Design review of the part built by this model. Coordinates are the model's own, in mm. A direction names the side the tool comes from. Round coordinates to 2 decimals unless told otherwise and drop trailing zeros. Loops run counter-clockwise (first coordinate to the right, second up) from the corner with the lowest first, then second, coordinate; pieces in that order, holes last. Notation, with made-up numbers: (51.25, 21) -> (103.25, 21) arc R21 ccw to (103.25, 39) -> close; hole circle Ø8 at (86.5, 81.5). An arc over 180 degrees is marked (long way). Write each question's results on one line, items separated by ' | '. Start each with the question number.
from build123d import *

# Parameters (mm, degrees)
ESQUISSE1_R                                = 1.4
BOSS_EXTRU_1_DEPTH                         = 6
ESQUISSE2_R                                = 3.25
ENL_V_MAT_EXTRU_1_DEPTH                    = 3
SYM_TRIE3_AT_THE_SECOND_PLANE_COPY_1_SKE_R = 3.25
SYM_TRIE3_AT_THE_SECOND_PLANE_COPY_1_DEPTH = 3
ESQUISSE4_W                                = 25
ESQUISSE4_H                                = 5
ESQUISSE4_W_2                              = 7.5
ESQUISSE4_H_2                              = 50
ENL_V_MAT_EXTRU_2_DEPTH                    = 102.655363655


with BuildPart() as part:
    # Esquisse1 → Boss.-Extru.1 (new body)
    with BuildSketch(Plane(origin=(0, 0, -27.5), x_dir=(-1, 0, 0), z_dir=(0, 0, -1))):
        Polygon((-2.565563678, -55.727752809), (62.179602326, -55.727752809), (84.807019324, -33.100335811), (84.807019324, 31.644830193), (62.179602326, 54.272247191), (-2.565563678, 54.272247191), (-25.192980676, 31.644830193), (-25.192980676, -33.100335811), align=None)
        with Locations((-9.63663149, 38.715898005)):
            Circle(ESQUISSE1_R, mode=Mode.SUBTRACT)
        with Locations((69.250670138, 38.715898005)):
            Circle(ESQUISSE1_R, mode=Mode.SUBTRACT)
        with Locations((69.250670138, -40.171403623)):
            Circle(ESQUISSE1_R, mode=Mode.SUBTRACT)
        with Locations((-9.63663149, -40.171403623)):
            Circle(ESQUISSE1_R, mode=Mode.SUBTRACT)
    extrude(amount=BOSS_EXTRU_1_DEPTH)

    # Esquisse2 → Enlèv. mat.-Extru.1 (cut)
    with BuildSketch(Plane(origin=(0, 0, -33.5), x_dir=(-1, 0, 0), z_dir=(0, 0, -1))):
        with Locations((69.250670138, 38.715898005)):
            Circle(ESQUISSE2_R)
    enl_v_mat_extru_1 = extrude(amount=-ENL_V_MAT_EXTRU_1_DEPTH, mode=Mode.SUBTRACT)

    # Symétrie3: Enlèv. mat.-Extru.1 across plane
    add(enl_v_mat_extru_1.mirror(Plane(origin=(-29.807019324, 0, 0), x_dir=(0, 0, 1), z_dir=(1, 0, 0))), mode=Mode.SUBTRACT)

    # Symétrie3 at the second plane: Enlèv. mat.-Extru.1 across plane
    add(enl_v_mat_extru_1.mirror(Plane(origin=(0, -0.727752809, 0), x_dir=(0, 0, 1), z_dir=(0, -1, 0))), mode=Mode.SUBTRACT)

    # Symétrie3 at the second plane copy 1 ske → Symétrie3 at the second plane copy 1 (cut)
    with BuildSketch(Plane(origin=(-59.614038648, -1.455505618, -33.5), x_dir=(1, 0, 0), z_dir=(0, 0, -1))):
        with Locations((69.250670138, 38.715898005)):
            Circle(SYM_TRIE3_AT_THE_SECOND_PLANE_COPY_1_SKE_R)
    extrude(amount=-SYM_TRIE3_AT_THE_SECOND_PLANE_COPY_1_DEPTH, mode=Mode.SUBTRACT)

    # Esquisse4 → Enlèv. mat.-Extru.2 (cut, through all)
    with BuildSketch(Plane(origin=(0, 0, -33.5), x_dir=(-1, 0, 0), z_dir=(0, 0, -1))):
        with Locations((39.250670138, -40.171403623)):
            Rectangle(ESQUISSE4_W, ESQUISSE4_H)
        with Locations((39.250670138, 38.715898005)):
            Rectangle(ESQUISSE4_W, ESQUISSE4_H)
        with Locations((-5.88663149, -0.727752809)):
            Rectangle(ESQUISSE4_W_2, ESQUISSE4_H_2)
    extrude(amount=-ENL_V_MAT_EXTRU_2_DEPTH, mode=Mode.SUBTRACT)


solid = part.part
1) Insertion check: pin 1 (7 mm diameter, centred on x = -70.5, y = -39.5, fed in from -Z); pin 2 (2.5 mm diameter, centred on x = -69.25, y = -40.17, fed in from +Z); pin 3 (2 mm diameter, centred on x = 9, y = -39, fed in from -Z); pin 4 (1.5 mm diameter, centred on y = 38, z = -30.5, fed in from -X). Each pin has a flat end and moves straight along its axis. Give the tip position at first contact, or say it passes through.
2) To check wall thickness, follow line 1 (Y direction, x = -32, z = -29.85); line 2 (X direction, y = 23, z = -31.6); line 3 (Y direction, x = -69, z = -31.1). State the ranges of each line that lie inside material, in increasing order. Write a range as from..to.
3) Take a section at A-A (y = 19). Write out the cut boundary in (x, z), plus the area to 3 significant figures.
4) For faces 4 (the face through (-39, -37.671, -31)), 5 (the face through (-72.35, -41.15, -32.02)), 6 (the face through (13.72, 43.12, -30.46)), list the 3-axis set-ups (+Z, -Z, +X, -X, +Y, -Y) from which the entire face can be reached by the end or side of a thin tool; tool diameter is ignored.
5) Take a section at C-C (z = -32.05). Write out the cut boundary in (x, y), plus the area to 3 significant figures.
6) The part is to be moulded in two halves that separate along X. For faces 1 (the face through (-51.751, -40, -31)), 2 (the face through (25.193, 0, -30)), 3 (the face through (-29, -55.728, -30)), say which applies: +X half, -X half, draft (parallel to the pull), parting line (faces both ways), or undercut.
7) Take a section at D-D (y = 45.5). Write out the cut boundary in (x, z), plus the area to 3 significant figures.
8) Take a section at B-B (x = -31). Write out the cut boundary in (y, z), plus the area to 3 significant figures.
Geometry check:
1) pin 1: stops at z = -33.5 | pin 2: passes through | pin 3: stops at z = -30.5 | pin 4: stops at x = -79.2
2) line 1: y = -55.73..-42.67, -37.67..36.22, 41.22..54.27 | line 2: x = -84.81..2.14, 9.64..25.19 | line 3: y = -48.91..-43.41, -36.93..35.48, 41.96..47.45
3) outline: (-84.81, -33.5) -> (2.14, -33.5) -> (2.14, -27.5) -> (-84.81, -27.5) -> close; (9.64, -33.5) -> (25.19, -33.5) -> (25.19, -27.5) -> (9.64, -27.5) -> close | area: 615 mm^2
4) face 4: +Z, -Z | face 5: -Z | face 6: +Z, -Z, +X, +Y
5) outline: (-84.81, -33.1) -> (-62.18, -55.73) -> (2.57, -55.73) -> (25.19, -33.1) -> (25.19, 31.64) -> (2.57, 54.27) -> (-62.18, 54.27) -> (-84.81, 31.64) -> close; hole circle Ø6.5 at (-69.25, -40.17); hole circle Ø6.5 at (-69.25, 38.72); hole (-51.75, -42.67) -> (-26.75, -42.67) -> (-26.75, -37.67) -> (-51.75, -37.67) -> close; hole (-51.75, 36.22) -> (-26.75, 36.22) -> (-26.75, 41.22) -> (-51.75, 41.22) -> close; hole (2.14, -25.73) -> (9.64, -25.73) -> (9.64, 24.27) -> (2.14, 24.27) -> close; hole circle Ø6.5 at (9.64, -40.17); hole circle Ø6.5 at (9.64, 38.72) | area: 10,300 mm^2
6) face 1: undercut | face 2: +X half | face 3: draft
7) outline: (-70.95, -33.5) -> (11.34, -33.5) -> (11.34, -27.5) -> (-70.95, -27.5) -> close | area: 494 mm^2
8) outline: (-55.73, -33.5) -> (-42.67, -33.5) -> (-42.67, -27.5) -> (-55.73, -27.5) -> close; (-37.67, -33.5) -> (36.22, -33.5) -> (36.22, -27.5) -> (-37.67, -27.5) -> close; (41.22, -33.5) -> (54.27, -33.5) -> (54.27, -27.5) -> (41.22, -27.5) -> close | area: 600 mm^2
